Part model, mm, in its own coordinate system. Coordinates: 2 decimals unless noted, no trailing zeros. Loops run counter-clockwise (first coordinate to the right, second up) from the corner with the lowest first, then second, coordinate; pieces in that order, holes last. Notation, with made-up numbers: (40.25, -1.5) - (88.25, -1.5) arc R31 cw to (88.25, 34.5) - close; hole circle Ø8 at (70.5, 82). An arc over 180 degrees is marked (long way). Use a Markdown table: item, result. Add a question column.
1. Wall check: probe 1 along Z at (x, y) = (297.5, 65.5); probe 2 along Y at (x, z) = (-104.5, -198); probe 3 along Z at (x, y) = (51.5, 51). Give the ranges that are in metal, low to high. Write a range as [from, to].
2. Band-saw the part on D-D, the plane x = -182. Give the cut face in (y, z).
3. Band-saw the part on B-B, the plane x = 514. Give the cut face in (y, z), plus the area to 3 significant figures.
4. Band-saw the part on A-A, the plane y = 94. Give the cut face in (x, z), plus the area to 3 significant figures.
5. Band-saw the part on C-C, the plane z = -412. Give the cut face in (x, y), plus the area to 3 significant figures.
6. Drop flat-ended pins along their axis: pin 1 (12.5 mm diameter, centred on x = 55.5, y = 66.5, fed in from +Z); pin 2 (15 mm diameter, centred on y = 49.5, z = 134, fed in from -X); pin 3 (20 mm diameter, centred on x = 84, y = 60.5, fed in from +Z). Give the stop position or say it passes through.
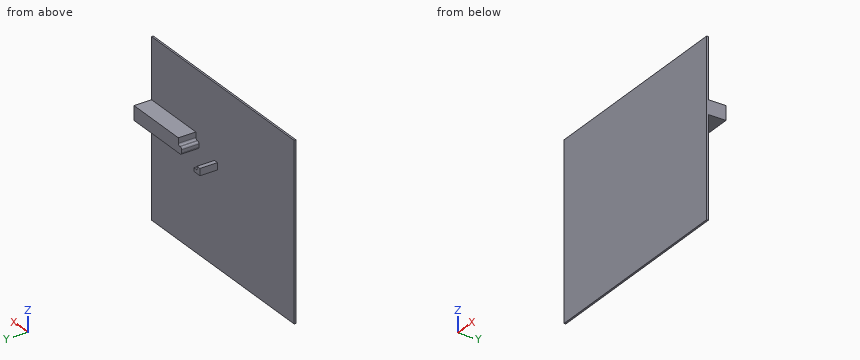
from build123d import *

# Parameters (mm, degrees)
SKETCH2_W           = 1200
SKETCH2_H           = 1000
BOSS_EXTRUDE1_DEPTH = 10
BOSS_EXTRUDE2_DEPTH = 100
BOSS_EXTRUDE3_DEPTH = 100


with BuildPart() as part:
    # Sketch2 → Boss-Extrude1 (new body)
    with BuildSketch(Plane(origin=(0, 0, 0), x_dir=(1, 0, 0), z_dir=(0, 1, 0))):
        Rectangle(SKETCH2_W, SKETCH2_H)
    extrude(amount=BOSS_EXTRUDE1_DEPTH)

    # Sketch4 → Boss-Extrude2 (add)
    with BuildSketch(Plane(origin=(0, 10, 0), x_dir=(1, 0, 0), z_dir=(0, 1, 0))):
        with BuildLine():
            Line((211.500312891, -115.173130931), (216.500312891, -115.173130931))
            ThreePointArc((216.500312891, -115.173130931), (224.278487484, -118.394956338), (227.500312891, -126.173130931))
            Line((227.500312891, -126.173130931), (227.500312891, -156.173130931))
            Line((227.500312891, -156.173130931), (600, -156.173130931))
            Line((600, -156.173130931), (600, -95.173130931))
            Line((600, -95.173130931), (600, -75.173130931))
            Line((600, -75.173130931), (211.500312891, -75.173130931))
            ThreePointArc((211.500312891, -75.173130931), (203.722138298, -78.394956338), (200.500312891, -86.173130931))
            Line((200.500312891, -86.173130931), (200.500312891, -104.173130931))
            ThreePointArc((200.500312891, -104.173130931), (203.722138298, -111.951305524), (211.500312891, -115.173130931))
        make_face()
    extrude(amount=BOSS_EXTRUDE2_DEPTH)

    # Sketch5 → Boss-Extrude3 (add)
    with BuildSketch(Plane(origin=(0, 10, 0), x_dir=(1, 0, 0), z_dir=(0, 1, 0))):
        Polygon((95.500312891, -55.173130931), (95.500312891, -35.173130931), (45.500312891, -35.173130931), (45.500312891, -75.173130931), (70.500312891, -75.173130931), (70.500312891, -55.173130931), align=None)
    extrude(amount=BOSS_EXTRUDE3_DEPTH)


solid = part.part
Geometry check:
| question | item | result |
|---|---|---|
| 1 | probe 1 | z = [75.17, 156.17] |
| 1 | probe 2 | y = [0, 10] |
| 1 | probe 3 | z = [35.17, 75.17] |
| 2 | outline | (0, -500) - (10, -500) - (10, 500) - (0, 500) - close |
| 3 | outline | (0, -500) - (10, -500) - (10, 75.17) - (110, 75.17) - (110, 156.17) - (10, 156.17) - (10, 500) - (0, 500) - close |
| 3 | area | 18,100 mm^2 |
| 4 | outline | (45.5, 35.17) - (95.5, 35.17) - (95.5, 55.17) - (70.5, 55.17) - (70.5, 75.17) - (45.5, 75.17) - close; (200.5, 86.17) arc R11 ccw to (211.5, 75.17) - (600, 75.17) - (600, 156.17) - (227.5, 156.17) - (227.5, 126.17) arc R11 cw to (216.5, 115.17) - (211.5, 115.17) arc R11 ccw to (200.5, 104.17) - close |
| 4 | area | 32,700 mm^2 |
| 5 | outline | (-600, 0) - (600, 0) - (600, 10) - (-600, 10) - close |
| 5 | area | 12,000 mm^2 |
| 6 | pin 1 | stops at z = 75.17 |
| 6 | pin 2 | stops at x = 227.5 |
| 6 | pin 3 | stops at z = 55.17 |
